```python
from build123d import *

# Parameters (mm, degrees)
SKETCH1_W           = 112
SKETCH1_H           = 176
SKETCH1_R           = 2.35
BOSS_EXTRUDE1_DEPTH = 2.54
FILLET1_R           = 8
SKETCH2_W           = 10
SKETCH2_H           = 144
CUT_EXTRUDE1_DEPTH  = 3.18
FILLET2_R           = 8
FILLET3_R           = 8


with BuildPart() as part:
    # Sketch1 → Boss-Extrude1 (new body)
    with BuildSketch(Plane.XY):
        Rectangle(SKETCH1_W, SKETCH1_H)
        with Locations((-48, 80)):
            Circle(SKETCH1_R, mode=Mode.SUBTRACT)
        with Locations((48, 80)):
            Circle(SKETCH1_R, mode=Mode.SUBTRACT)
        with Locations((48, -80)):
            Circle(SKETCH1_R, mode=Mode.SUBTRACT)
        with Locations((-48, -80)):
            Circle(SKETCH1_R, mode=Mode.SUBTRACT)
    extrude(amount=BOSS_EXTRUDE1_DEPTH)

    # Fillet1
    fillet1_edges = [part.edges().sort_by_distance(p)[0] for p in [
        (56, -88, 1.27),
        (-56, -88, 1.27),
        (-56, 88, 1.27),
        (56, 88, 1.27),
    ]]
    fillet(fillet1_edges, radius=FILLET1_R)

    # Sketch2 → Cut-Extrude1 (cut)
    with BuildSketch(Plane.XY.offset(2.54)):
        with Locations((-51, 0)):
            Rectangle(SKETCH2_W, SKETCH2_H)
        with Locations((51, 0)):
            Rectangle(SKETCH2_W, SKETCH2_H)
    extrude(amount=-CUT_EXTRUDE1_DEPTH, mode=Mode.SUBTRACT)

    # Fillet2
    fillet2_edges = [part.edges().sort_by_distance(p)[0] for p in [
        (56, 72, 1.27),
        (56, -72, 1.27),
        (-56, -72, 1.27),
        (-56, 72, 1.27),
    ]]
    fillet(fillet2_edges, radius=FILLET2_R - 0.0001)  # a hair under: the kernel refuses the full size

    # Fillet3
    fillet3_edges = [part.edges().sort_by_distance(p)[0] for p in [
        (46, -72, 1.27),
        (46, 72, 1.27),
        (-46, 72, 1.27),
        (-46, -72, 1.27),
    ]]
    fillet(fillet3_edges, radius=FILLET3_R)


solid = part.part
```
Geometry: final body of the model. Coordinates: model frame, mm. A direction names the side the tool comes from. Round coordinates to 2 decimals unless told otherwise and drop trailing zeros. Loops run counter-clockwise (first coordinate to the right, second up) from the corner with the lowest first, then second, coordinate; pieces in that order, holes last.
Item 1: Mould query, pull axis Y, two halves, no side actions, for faces 1 (the cylindrical face through (-53.719, -85.594, 1.288)), 2 (the cylindrical face through (-53.719, 85.594, 1.288)), 3 (the flat face through (-1, 1, 0)), 4 (the cylindrical face through (-46.737, 81.982, 1.252)). Classes: released by +Y, released by -Y, zero draft, split by the parting line, or undercut.
Checked values:
face 1: released by -Y
face 2: released by +Y
face 3: zero draft
face 4: undercut
Item 2: Reachability of faces 5 (the cylindrical face through (-46.737, -78.018, 1.252)), 6 (the cylindrical face through (54.596, -75.473, 1.252)), 7 (the cylindrical face through (-54.67, -75.58, 1.25)) from +Z, -Z, +X, -X, +Y, -Y: full face, straight path, thin tool, end or side. Return the list, or none.
Checked values:
face 5: +Z, -Z
face 6: +Z, -Z, +X
face 7: +Z, -Z, -X
Item 3: Section B-B, the plane z = 1.35. State how many separate pieces and enclosed holes the cut face has, plus the area to 3 significant figures.
Checked values:
separate pieces: 1
enclosed holes: 4
area: 16,700 mm2
Item 4: Contact query for flat-ended pins moving along their axis: P1, Ø6, axis at x = 48, y = -80, coming from the +Z side; P2, Ø1.3, axis at y = -2.5, z = 1, coming from the -X side; P3, Ø4, axis at x = -48, y = 80, coming from the +Z side; P4, Ø1, axis at y = -50, z = 1.5, coming from the +X side. Output: stop coordinate, or through.
Checked values:
P1: stops at z = 2.54
P2: stops at x = -46
P3: passes through
P4: stops at x = 46
Item 5: Line query: L1, parallel to Y at x = 48, z = 1.5; L2, parallel to X at y = -41, z = 0.35; L3, parallel to X at y = -67, z = 0.6. Output: solid intervals per line, ascending.
Checked values:
L1: y = -88 to -82.35, -77.65 to -70.46, 70.46 to 77.65, 82.35 to 88
L2: x = -46 to 46
L3: x = -46.21 to 46.21
Item 6: Section A-A, the plane y = -31. Output: boundary loops of the cut face in (x, z).
Checked values:
outline: (-46, 0) - (46, 0) - (46, 2.54) - (-46, 2.54) - close
